Build history of the part. All positions in model axes, mm. A direction names the side the tool comes from. Round coordinates to 2 decimals unless told otherwise and drop trailing zeros. Order: outer loops, then holes, each group sorted by start corner. A loop starts at its lowest first (then second) coordinate and runs counter-clockwise, first axis right, second up. Notation, with made-up numbers: (12.5, 81) -> (53.5, 81) arc R20 cw to (53.5, 119) -> close; hole circle Ø5 at (45, -11). An arc over 180 degrees is marked (long way). Write item = value, one per line.
from build123d import *

# Parameters (mm, degrees)
F0_W     = 50.8
F0_H     = 31.75
F1_DEPTH = 31.75
F2_W     = 19.05
F2_H     = 19.05
F3_DEPTH = 19.05
F4_W     = 19.05
F4_H     = 19.05
F5_DEPTH = 19.05
F7_DEPTH = 12.7
F9_DEPTH = 12.7


with BuildPart() as f1:
    # F0 (on Front) → F1 (new body)
    with BuildSketch(Plane.XZ):
        with Locations((25.4, 15.875)):
            Rectangle(F0_W, F0_H)
    extrude(amount=F1_DEPTH)

    # F2 (on face) → F3 (cut)
    with BuildSketch(Plane.YZ.offset(50.8)):
        with Locations((-22.225, 22.225)):
            Rectangle(F2_W, F2_H)
    extrude(amount=-F3_DEPTH, mode=Mode.SUBTRACT)

    # F4 (on face) → F5 (cut)
    with BuildSketch(Plane(origin=(0, 0, 0), x_dir=(0, -1, 0), z_dir=(-1, 0, 0))):
        with Locations((22.225, 22.225)):
            Rectangle(F4_W, F4_H)
    extrude(amount=-F5_DEPTH, mode=Mode.SUBTRACT)

    # F6 (on face) → F7 (cut)
    with BuildSketch(Plane.XZ.offset(12.7)):
        Polygon((50.8, 31.75), (41.275, 31.75), (50.8, 12.7), align=None)
    extrude(amount=-F7_DEPTH, mode=Mode.SUBTRACT)

    # F8 (on face) → F9 (cut)
    with BuildSketch(Plane.YZ.offset(31.75)):
        Polygon((-31.75, 12.7), (-12.7, 31.75), (-31.75, 31.75), align=None)
    extrude(amount=-F9_DEPTH, mode=Mode.SUBTRACT)


solid = f1.part
Q1. Cut at C-C, the plane x = 5. List the corners of the cut face in (y, z).
Check values:
outline = (-31.75, 0) -> (0, 0) -> (0, 31.75) -> (-12.7, 31.75) -> (-12.7, 12.7) -> (-31.75, 12.7) -> close
Q2. Cut at B-B, the plane y = -9.5. List the corners of the cut face in (x, z) (3 decimals).
Check values:
outline = (0, 0) -> (50.8, 0) -> (50.8, 12.7) -> (41.275, 31.75) -> (0, 31.75) -> close
Q3. Probe probe 1 along Y at (x, z) = (8, 28.5); probe 2 along X at (y, z) = (-27.5, 15); probe 3 along Z at (x, y) = (7.5, -22.5). List the from-to ranges inside material, lowest first.
Check values:
probe_1 = -12.7 to 0
probe_2 = 19.05 to 31.75
probe_3 = 0 to 12.7
Q4. Which spindle directions (+Z, -Z, +X, -X, +Y, -Y) get a long thin tool onto all of the face, cutting with end or side? Do faces 1 (the face through (0, -12, 12)), 2 (the face through (39, -12.7, 22)), 3 (the face through (19.05, -18, 18)). Say none if no direction does.
Check values:
face_1 = +Z, -Z, -X, +Y, -Y
face_2 = +Z, +X, -Y
face_3 = +Z, -X, -Y
Q5. Cut at A-A, the plane z = 28. List the corners of the cut face in (x, y), and give its area (3 significant figures).
Check values:
outline = (0, -12.7) -> (19.05, -12.7) -> (19.05, -16.45) -> (31.75, -16.45) -> (31.75, -12.7) -> (43.15, -12.7) -> (43.15, 0) -> (0, 0) -> close
area = 596 mm²
Q6. Cut at D-D, the plane z = 21. List the corners of the cut face in (x, y), and give its area (3 significant figures).
Check values:
outline = (0, -12.7) -> (19.05, -12.7) -> (19.05, -23.45) -> (31.75, -23.45) -> (31.75, -12.7) -> (46.65, -12.7) -> (46.65, 0) -> (0, 0) -> close
area = 729 mm²
Q7. Flat gauge pins, fed straight in: pin 1 (5.5 mm diameter, centred on x = 42.5, y = -20, fed in from +Z); pin 2 (15 mm diameter, centred on x = 44, z = 23.5, fed in from -Y); pin 3 (15 mm diameter, centred on y = -25, z = 24.5, fed in from +X). Where does each tip first touch, or does it go through?
Check values:
pin_1 = 12.7
pin_2 = -12.7
pin_3 = 31.75
